Autodesk Inventor part; units mm, degrees
ref_plane "YZ Plane" through (0, 0, 0) normal (1, 0, 0) x (0, 1, 0)
ref_plane "XZ Plane" through (0, 0, 0) normal (0, 1, 0) x (-1, 0, 0)
ref_plane "XY Plane" through (0, 0, 0) normal (0, 0, 1) x (1, 0, 0)
sketch "Skizze1" plane through (0, 0, 0) normal (0, 1, 0) x (-1, 0, 0)
  line L0 (-15, -97) -> (15, -97)
  line L1 (20, -92) -> (20, 92)
  line L2 (15, 97) -> (-15, 97)
  line L3 (-20, 92) -> (-20, -92)
  line L4 (-20, -97) -> (20, 97) construction
  line L5 (20, -97) -> (-20, 97) construction
  arc A0 (20, 95) -> (18, 97) centre (18, 95) ccw
  arc A1 (20, 92) -> (15, 97) centre (15, 92) ccw
  arc A2 (-15, 97) -> (-20, 92) centre (-15, 92) ccw
  arc A3 (-20, -92) -> (-15, -97) centre (-15, -92) ccw
  arc A4 (15, -97) -> (20, -92) centre (15, -92) ccw
  point P0 (0, 0)
  dimension "d0" = 40
  dimension "d1" = 194
  dimension "d3" = 5
  dimension "d4" = 5
extrude "Extrusion1" add sketch "Skizze1" along normal blind 55
sketch "Skizze2" plane through (0, 0, 0) normal (0, -1, 0) x (1, 0, 0)
  circle A0 centre (0, 82) radius 4.188
  line L0 (-15, 97) -> (15, 97)
  point P0 (0, 0)
  dimension "d7" = 8.376
  dimension "d8" = 15
extrude "Extrusion2" add sketch "Skizze2" along normal blind 18
fillet "Rundung1" radius 5 8 edges at (18.5355, 0, 95.5355) (20, 0, 0) (18.5355, 0, -95.5355) (0, 0, -97) (-18.5355, 0, -95.5355) (-20, 0, 0) (-18.5355, 0, 95.5355) (0, 0, 97)
properties part number "Schmierung" material "Wasser"
Input: part model. Units: mm. Frame: model coordinates. A direction names the side the tool comes from. Give positions to 0.01 mm unless a question says otherwise; leave off trailing zeros. Write each loop counter-clockwise with the first axis right and the second up, starting at its lowest first coordinate (ties: lowest second). Pieces come first, ordered by that corner, then holes. Notation, with made-up numbers: (-28.5, 8) - (2.5, 8) arc R36 ccw to (2.5, 44) - close; hole circle Ø11 at (10.5, -5). An arc over 180 degrees is marked (long way). Write item = value, one per line. Start each with the question number.
1. Section query C-C, the plane y = -10. Output: boundary loops of the cut face in (x, z), then the cut area to 3 significant figures.
2. First-contact query: pin 1 Ø1 at (x, y) = (4.5, 1) entering from -Z; pin 2 Ø3 at (x, z) = (-7.5, 50) entering from -Y; pin 3 Ø5 at (x, y) = (-1.5, -5.5) entering from +Z. Flat tips, straight axial feed; report the tip coordinate or a pass-through.
3. Section query B-B, the plane x = 0. Output: boundary loops of the cut face in (y, z).
4. Section query A-A, the plane z = 82. Output: boundary loops of the cut face in (x, y), then the cut area to 3 significant figures.
5. Section query D-D, the plane x = -17. Output: boundary loops of the cut face in (y, z), then the cut area to 3 significant figures.
6. Access query for faces 1 (the cylindrical face through (-0.55, -8.87, 77.85)), 2 (the flat face through (0, 55, 1)). Directions: +Z, -Z, +X, -X, +Y, -Y. A direction counts if a zero-diameter tool reaches every point of the face in a straight line with its end or side. Return the directions, or none.
7. Ray query, L1, parallel to Z at x = 0, y = -10.5; L2, parallel to Y at x = 7, z = -21; L3, parallel to Z at x = 3, y = -6.5. Return the intervals inside material, ascending.
Check sheet entries:
q1.outline = circle Ø8.38 at (0, 82)
q1.area = 55.1 mm2
q2.pin_1 = -95.57
q2.pin_2 = 0
q2.pin_3 = 86.19
q3.outline = (-18, 77.81) - (0, 77.81) - (0, -92) arc R5 ccw to (5, -97) - (55, -97) - (55, 97) - (5, 97) arc R5 ccw to (0, 92) - (0, 86.19) - (-18, 86.19) - close
q4.outline = (-20, 5) arc R5 ccw to (-15, 0) - (-4.19, 0) - (-4.19, -18) - (4.19, -18) - (4.19, 0) - (15, 0) arc R5 ccw to (20, 5) - (20, 55) - (-20, 55) - close
q4.area = 2,340 mm2
q5.outline = (0.42, -92) arc R4.58 ccw to (5, -96.58) - (55, -96.58) - (55, 96.58) - (5, 96.58) arc R4.58 ccw to (0.42, 92) - close
q5.area = 10,500 mm2
q6.face_1 = -Y
q6.face_2 = +Z, -Z, +X, -X, +Y
q7.L1 = 77.81 to 86.19
q7.L2 = 0 to 55
q7.L3 = 79.08 to 84.92
